Can you work these out from the model? Positions are in its coordinate system, mm. Round coordinates to 2 decimals unless told otherwise and drop trailing zeros. Order: outer loops, then holes, each group sorted by start corner. A loop starts at its lowest first (then second) coordinate and runs counter-clockwise, first axis right, second up.
Q1. If I drill on line 1 (X direction, y = 208, z = 3.75); line 2 (Y direction, x = 0, z = 12.5); line 3 (X direction, y = 10, z = 17), over which ranges is the centre line in solid material (lowest first)?
Q2. If we section it at A-A (x = 0): Please give me the cut outline in (y, z).
Q3. If we section it at B-B (z = 4.75): Please give me the cut outline in (x, y).
Q4. Will these pins go through, and if not, where does the flat tip stop? P1, Ø3, axis at y = 120, z = 7.5, coming from the -X side; P2, Ø2, axis at x = 0.5, z = 8, coming from the -Y side.
Q5. We'd pull the mould along X, two halves only. Please class faces 1 (the face through (0, 3, 19.05)), 2 (the face through (-20.307, -0.737, 9.392)), 3 (the face through (20.32, 111, 9)): pulls with the +X half, pulls with the -X half, needs draft (parallel to the pull), parting line crosses it, or undercut.
from build123d import *

# Parameters (mm, degrees)
EXTRUDE1_DEPTH     = 19.05
SKETCH2_R          = 2.38125
CUT_EXTRUDE1_DEPTH = 0.254


with BuildPart() as part:
    # Sketch1 → Extrude1 (new body)
    with BuildSketch(Plane.XY):
        with BuildLine():
            Line((20.32, 0), (20.32, 226.06))
            Line((20.32, 226.06), (20.066, 226.06))
            Line((20.066, 226.06), (20.066, 3.202818134))
            ThreePointArc((20.066, 3.202818134), (-20.25640047, -1.606437051), (20.32, 0))
        make_face()
    extrude(amount=EXTRUDE1_DEPTH)

    # Sketch2 → Cut-Extrude1 (cut)
    with BuildSketch(Plane(origin=(20.32, 0, 0), x_dir=(0, 0, -1), z_dir=(1, 0, 0))):
        with Locations(Location((-9.525, 218.1225, 0), (0, 0, 90))):
            Circle(SKETCH2_R)
    extrude(amount=-CUT_EXTRUDE1_DEPTH, mode=Mode.SUBTRACT)


solid = part.part
Solution:
1. line 1: x = 20.07 to 20.32
1. line 2: y = -20.32 to 20.32
1. line 3: x = -17.69 to 17.69, 20.07 to 20.32
2. outline: (-20.32, 0) - (20.32, 0) - (20.32, 19.05) - (-20.32, 19.05) - close
3. outline: (20.07, 3.2) arc R20.32 ccw (long way) to (20.32, 0) - (20.32, 226.06) - (20.07, 226.06) - close
4. P1: stops at x = 20.07
4. P2: stops at y = -20.32
5. face 1: needs draft
5. face 2: undercut
5. face 3: pulls with the +X half
